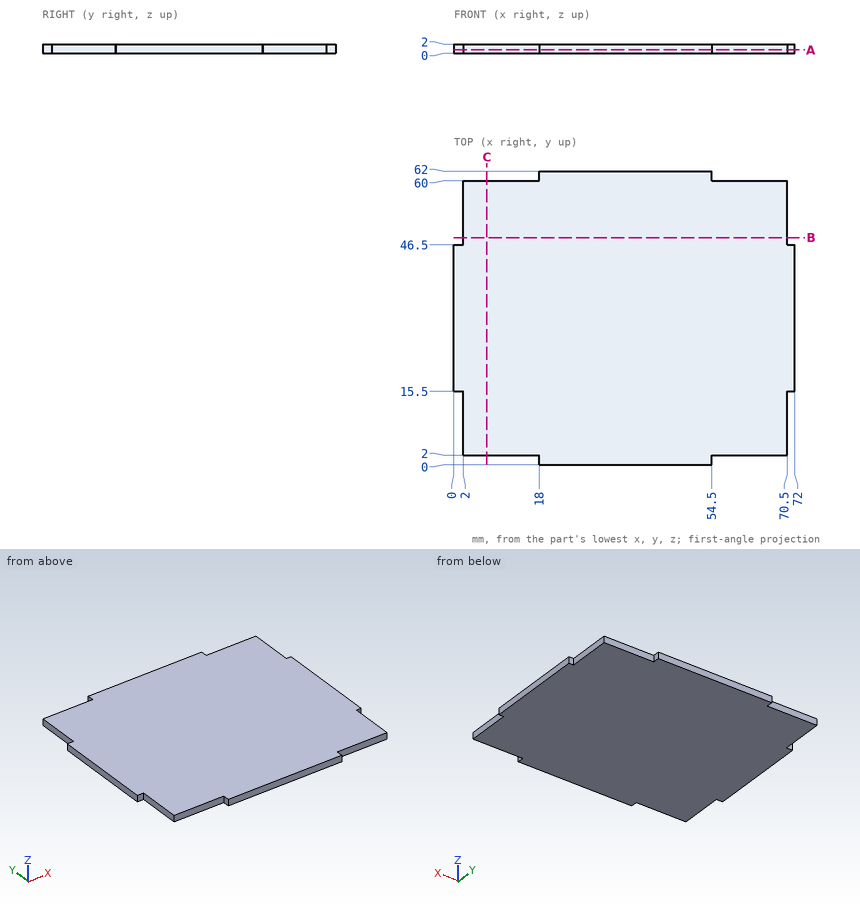
Study the drawing (mm; zero at the part's minimum x, y, z) and answer. Coordinates: 2 decimals unless noted, no trailing zeros. Loops run counter-clockwise (first coordinate to the right, second up) from the corner with the lowest first, then second, coordinate; pieces in that order, holes last. Notation, with made-up numbers: M -30,66.25 L 29,66.25 A22 ccw 29,98.25 Z; hole C 85,86.25 d1. An arc over 180 degrees is marked long. Answer as a JSON object with one key per item and string values. Group by question number.
Item 1: Section B-B (y = 48) is taken. Write down the section's boundary in (x, z), and give its area (3 significant figures).
Item 2: Section C-C (x = 7) is taken. Write down the section's boundary in (y, z).
Item 3: Section A-A (z = 0.75) is taken. Write down the section's boundary in (x, y).
Item 4: Consider L1, parallel to Y at x = 64, z = 0.35; L2, parallel to X at y = 50, z = 1.4. Determine where each line is inside the solid, lowest interval first.
Item 5: Each of these flat-tipped pins is pushed along its axis until it touches: P1, Ø0.6, axis at y = 9.5, z = 0.5, coming from the -X side; P2, Ø1, axis at x = 1, z = 1.5, coming from the -Y side; P3, Ø0.6, axis at y = 61.5, z = 1.5, coming from the +X side; P4, Ø10, axis at x = 40.5, y = 25.5, coming from the -Z side. Where does it stop, or does it pass through?
Solved:
{
 "1": {"outline": "M 2,0 L 70.5,0 L 70.5,2 L 2,2 Z", "area": "137 mm2"},
 "2": {"outline": "M 2,0 L 60,0 L 60,2 L 2,2 Z"},
 "3": {"outline": "M 0,15.5 L 2,15.5 L 2,2 L 18,2 L 18,0 L 54.5,0 L 54.5,2 L 70.5,2 L 70.5,15.5 L 72,15.5 L 72,46.5 L 70.5,46.5 L 70.5,60 L 54.5,60 L 54.5,62 L 18,62 L 18,60 L 2,60 L 2,46.5 L 0,46.5 Z"},
 "4": {"L1": "y = 2 to 60", "L2": "x = 2 to 70.5"},
 "5": {"P1": "stops at x = 2", "P2": "stops at y = 15.5", "P3": "stops at x = 54.5", "P4": "stops at z = 0"}
}
